Check sheet for the modelled part. Datum: model origin and axes. Units: mm. A direction names the side the tool comes from. Coordinates: 2 decimals unless noted, no trailing zeros. Loops run counter-clockwise (first coordinate to the right, second up) from the corner with the lowest first, then second, coordinate; pieces in that order, holes last. Notation, with made-up numbers: (-13.5, -25.5) -> (6.5, -25.5) arc R12 cw to (6.5, -10.5) -> close; hole circle Ø8 at (-36, 14.25). An arc over 180 degrees is marked (long way). Use one line per item in the form item = value.
Autodesk Fusion 360 part; units mm, degrees
sketch "Sketch1" plane through (0, 0, 0) normal (0, 0, 1) x (1, 0, 0)
  line L0 (0, 0) -> (150, 0)
  line L1 (0, 0) -> (0, 55)
  line L2 (35, 90) -> (115, 90)
  line L3 (150, 55) -> (150, 0)
  line L4 (0, 55) -> (35, 90)
  line L5 (150, 55) -> (115, 90)
  point P0 (0, 90)
  point P1 (150, 90)
  dimension "d1" = 150
  dimension "d2" = 90
  dimension "d3" = 35
  dimension "d4" = 35
  dimension "d5" = 35
  dimension "d6" = 35
extrude "Extrude1" add sketch "Sketch1" along normal mid plane 12
sketch "Sketch2" plane through (0, 0, 6) normal (0, 0, 1) x (1, 0, 0)
  line L0 (0, 0) -> (150, 0)
  line L1 (150, 0) -> (150, 55)
  line L2 (150, 55) -> (115, 90)
  line L3 (115, 90) -> (35, 90)
  line L4 (35, 90) -> (0, 55)
  line L5 (0, 55) -> (0, 0)
  line L6 (0, 12) -> (150, 12)
  line L7 (150, 0) -> (0, 0)
  dimension "d9" = 12
extrude "Extrude2" add sketch "Sketch2" along normal blind 40 contours L0 L1 L5 L6 L7
sketch "Sketch3" plane through (0, 12, 0) normal (0, 1, 0) x (-1, 0, 0)
  line L0 (-150, 6) -> (0, 6)
  line L1 (0, 6) -> (0, 46)
  line L2 (0, 46) -> (-150, 46)
  line L3 (-150, 46) -> (-150, 6)
  line L4 (0, 46) -> (-75, 71)
  line L5 (-75, 71) -> (-150, 46)
  line L6 (-75, 11.1392) -> (-75, 80.8608)
  dimension "d12" = 25
  dimension "d13" = 25
extrude "Extrude3" add sketch "Sketch3" against normal blind 12 contours L2 L5 L6 | L2 L4 L6
sketch "Sketch4" plane through (0, 0, 6) normal (0, 0, 1) x (1, 0, 0)
  line L0 (0, 12) -> (150, 12)
  line L1 (150, 12) -> (150, 55)
  line L2 (150, 55) -> (115, 90)
  line L3 (115, 90) -> (35, 90)
  line L4 (35, 90) -> (0, 55)
  line L5 (0, 55) -> (0, 12)
sketch "Sketch5" plane through (0, 0, 0) normal (1, 0, 0) x (0, 0, -1)
extrude "Extrude4" add sketch "Sketch3" along normal blind 30 contours L2 L5 L6 | L2 L4 L6
(1) Scan lines: line 1 along Y through (x, z) = (136.5, 44.5); line 2 along Z through (x, y) = (34, 79); line 3 along Y through (x, z) = (25, 50). Record each from-to range of solid material in increasing order.
Established:
line_1 = 0 to 12
line_2 = -6 to 6
line_3 = 0 to 42
(2) Go/stop test with flat-tipped pins: P1, Ø2, axis at x = 31.5, y = 52.5, coming from the +Z side; P2, Ø10, axis at x = 87, z = 24.5, coming from the +Y side; P3, Ø10, axis at x = 57, z = 60, coming from the +Y side; P4, Ø1.5, axis at y = 72, z = 8.5, coming from the +X side. Record where each tip stops, or that it passes through.
Established:
P1 = 6
P2 = 12
P3 = 42
P4 = through
(3) Section check A-A, the plane y = 15.5. Record the boundary of the cut face in (x, z), plus the area to 4 significant figures.
Established:
outline = (0, -6) -> (150, -6) -> (150, 6) -> (0, 6) -> close; (0, 46) -> (150, 46) -> (75, 71) -> close
area = 3,675 mm²
(4) Mould release check, pull along Z, two halves, no side actions. Record for faces 4 (the flat face through (36.975, 21.294, 58.325)), 5 (the flat face through (74, 12, 26)), 6 (the flat face through (74, 46, -6)), 7 (the flat face through (150, 15, 2)): +Z half, -Z half, draft (parallel to the pull), parting line (faces both ways), or undercut.
Established:
face_4 = +Z half
face_5 = undercut
face_6 = -Z half
face_7 = draft
(5) Tool access check on faces 1 (the flat face through (74, 27, 46)), 2 (the flat face through (76, 42, 56)), 3 (the flat face through (74, 90, 0)). Record the directions out of +Z, -Z, +X, -X, +Y, -Y that give a thin tool (end or side, any length) a straight path to the whole face; none if there is none.
Established:
face_1 = +X, -X, +Y
face_2 = +Z, +X, -X, +Y
face_3 = +Z, -Z, +X, -X, +Y
(6) Section check D-D, the plane y = 84.5. Record the boundary of the cut face in (x, z).
Established:
outline = (29.5, -6) -> (120.5, -6) -> (120.5, 6) -> (29.5, 6) -> close
(7) Section check B-B, the plane x = 124.5. Record the boundary of the cut face in (y, z).
Established:
outline = (0, -6) -> (80.5, -6) -> (80.5, 6) -> (12, 6) -> (12, 46) -> (42, 46) -> (42, 54.5) -> (0, 54.5) -> close
(8) Section check C-C, the plane z = 49. Record the boundary of the cut face in (x, y).
Established:
outline = (9, 0) -> (141, 0) -> (141, 42) -> (9, 42) -> close
